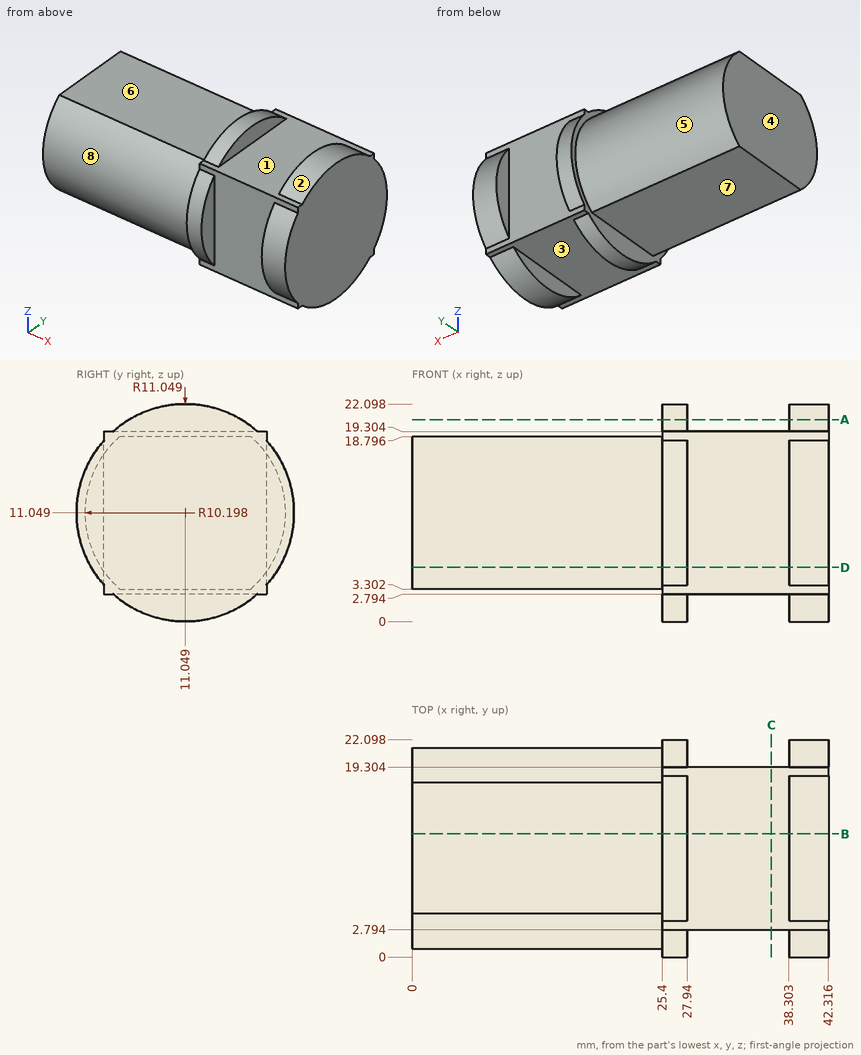
Part print with two shaded views. Sizes in mm from the minimum x, y, z corner. A direction names the side the tool comes from. Coordinates: 2 decimals unless noted, no trailing zeros. Write each loop counter-clockwise with the first axis right and the second up, starting at its lowest first coordinate (ties: lowest second). Pieces come first, ordered by that corner, then holes. Notation, with made-up numbers: (-11.75, 12) - (7.25, 12) arc R21 cw to (7.25, 47) - close; hole circle Ø9 at (7.25, 1.5). An arc over 180 degrees is marked (long way). Use a Markdown table: item, result. Add a question column.
Item 1: Drop flat-ended pins along their axis: pin 1 (8.5 mm diameter, centred on x = 33, y = 9.5, fed in from +Z); pin 2 (2 mm diameter, centred on x = 6.5, y = 5, fed in from +Z); pin 3 (2 mm diameter, centred on y = 11.5, z = 1.5, fed in from -X). Give the stop position or say it passes through.
Item 2: Drill centre lines: line 1 along X through (y, z) = (5.5, 2); line 2 along X through (y, z) = (20.5, 14); line 3 along Y through (x, z) = (32, 10.5). Where is each one in solid material? Low to high.
Item 3: Two-plate mould, pull along X, no slides. Class the marked faces 1, 2, 3 and 4: pulls with the +X half, pulls with the -X half, needs draft (parallel to the pull), parting line crosses it, or undercut.
Item 4: Band-saw the part on D-D, the plane z = 5.5. Write the cut outline in (x, y) (1 decimal), and give its area (3 significant figures).
Item 5: Band-saw the part on B-B, the plane y = 12.5. Write the cut outline in (x, z) (1 decimal).
Item 6: Band-saw the part on A-A, the plane z = 20.5. Write the cut outline in (x, y) (1 decimal).
Item 7: 3-axis set-ups, long thin cutter, end or side, ignore diameter. For the marked faces 5, 6, 7 and 8: which of +Z, -Z, +X, -X, +Y, -Y reach the whole face in a straight line?
Item 8: Band-saw the part on C-C, the plane x = 36.5. Write the cut outline in (y, z), and give its area (3 significant figures).
A:
| question | item | result |
|---|---|---|
| 1 | pin 1 | stops at z = 19.3 |
| 1 | pin 2 | stops at z = 18.8 |
| 1 | pin 3 | stops at x = 25.4 |
| 2 | line 1 | x = 25.4 to 27.94, 38.3 to 42.32 |
| 2 | line 2 | x = 0 to 27.94, 38.3 to 42.32 |
| 2 | line 3 | y = 2.79 to 19.3 |
| 3 | face 1 | undercut |
| 3 | face 2 | needs draft |
| 3 | face 3 | undercut |
| 3 | face 4 | pulls with the -X half |
| 4 | outline | (0, 2.5) - (25.4, 2.5) - (25.4, 1.5) - (27.9, 1.5) - (27.9, 2.8) - (38.3, 2.8) - (38.3, 1.5) - (42.3, 1.5) - (42.3, 20.6) - (38.3, 20.6) - (38.3, 19.3) - (27.9, 19.3) - (27.9, 20.6) - (25.4, 20.6) - (25.4, 19.6) - (0, 19.6) - close |
| 4 | area | 731 mm² |
| 5 | outline | (0, 3.3) - (25.4, 3.3) - (25.4, 0.1) - (27.9, 0.1) - (27.9, 2.8) - (38.3, 2.8) - (38.3, 0.1) - (42.3, 0.1) - (42.3, 22) - (38.3, 22) - (38.3, 19.3) - (27.9, 19.3) - (27.9, 22) - (25.4, 22) - (25.4, 18.8) - (0, 18.8) - close |
| 6 | outline | (25.4, 5.3) - (27.9, 5.3) - (27.9, 16.8) - (25.4, 16.8) - close; (38.3, 5.3) - (42.3, 5.3) - (42.3, 16.8) - (38.3, 16.8) - close |
| 7 | face 5 | -X, +Y |
| 7 | face 6 | +Z, -X, +Y, -Y |
| 7 | face 7 | -Z, -X, +Y, -Y |
| 7 | face 8 | -X, -Y |
| 8 | outline | (2.79, 2.79) - (19.3, 2.79) - (19.3, 19.3) - (2.79, 19.3) - close |
| 8 | area | 273 mm² |
